from build123d import *

# Parameters (mm, degrees)
SKETCH2_R           = 7.692100041
CUT_EXTRUDE1_DEPTH  = 10
SKETCH4_W           = 16.725751486
SKETCH4_H           = 29.132579912
BOSS_EXTRUDE1_DEPTH = 15
BOSS_EXTRUDE2_START = -29.132579912
BOSS_EXTRUDE2_DEPTH = 29.132579912
CUT_EXTRUDE2_DEPTH  = 72.857514692


with BuildPart() as part:
    # Sketch1 → Revolve1 (revolve)
    with BuildSketch(Plane(origin=(0, 0, 0), x_dir=(0, 0, -1), z_dir=(1, 0, 0)), mode=Mode.PRIVATE) as revolve1_sk:
        Polygon((18, 19), (53, 19), (53, 0), (56.096816333, 0), (56.096816333, 23.355709418), (18, 23.355709418), align=None)
    revolve(revolve1_sk.sketch.rotate(Axis((0, 0, -53), (0, 0, -1)), 90), axis=Axis((0, 0, -53), (0, 0, -1)))

    # Sketch2 → Cut-Extrude1 (cut)
    with BuildSketch(Plane(origin=(0, 0, -56.096816333), x_dir=(-1, 0, 0), z_dir=(0, 0, -1))):
        Circle(SKETCH2_R)
    extrude(amount=-CUT_EXTRUDE1_DEPTH, mode=Mode.SUBTRACT)



with BuildPart() as body_2:
    # Sketch4 → Boss-Extrude1 (new body)
    with BuildSketch(Plane(origin=(0, 23.355709418, 0), x_dir=(1, 0, 0), z_dir=(0, 1, 0))):
        with Locations((0, 36.155071486)):
            Rectangle(SKETCH4_W, SKETCH4_H)
    extrude(amount=BOSS_EXTRUDE1_DEPTH)


with BuildPart() as part_1:
    add(part.part)

    add(body_2.part)  # Boss-Extrude2 merges body 2
    # Sketch5 → Boss-Extrude2 (add)
    with BuildSketch(Plane(origin=(0, 0, -50.721361442), x_dir=(-1, 0, 0), z_dir=(0, 0, -1)).offset(BOSS_EXTRUDE2_START)):
        with BuildLine():
            ThreePointArc((-15.215762233, 17.71919135), (-8.113102925, 21.901295016), (0, 23.355709418))
            Line((0, 23.355709418), (-8.362875743, 23.355709418))
            Line((-8.362875743, 23.355709418), (-9.850694039, 23.211289977))
            add(Edge.make_bspline(
                [(-9.850694039, 23.211289977), (-13.176863257, 20.945911476), (-15.215762233, 17.71919135)],
                knots=[0, 0, 0, 0.793491279, 0.793491279, 0.793491279], degree=2))
        make_face()
        with BuildLine():
            add(Edge.make_bspline(
                [(9.850694039, 23.211289977), (13.176863257, 20.945911476), (15.215762233, 17.71919135)],
                knots=[0, 0, 0, 0.793491279, 0.793491279, 0.793491279], degree=2))
            Line((9.850694039, 23.211289977), (8.362875743, 23.355709418))
            Line((8.362875743, 23.355709418), (0, 23.355709418))
            ThreePointArc((0, 23.355709418), (8.113102925, 21.901295016), (15.215762233, 17.71919135))
        make_face()
    extrude(amount=BOSS_EXTRUDE2_DEPTH)

    # Sketch6 → Cut-Extrude2 (cut, through all)
    with BuildSketch(Plane.XY):
        with BuildLine():
            Line((-16.155494421, -10), (-21.106614187, -10))
            ThreePointArc((-21.106614187, -10), (-23.355709418, 0), (-21.106614187, 10))
            Line((-21.106614187, 10), (-16.155494421, 10))
            ThreePointArc((-16.155494421, 10), (-19, 0), (-16.155494421, -10))
        make_face()
    extrude(amount=-CUT_EXTRUDE2_DEPTH, mode=Mode.SUBTRACT)


solid = part_1.part
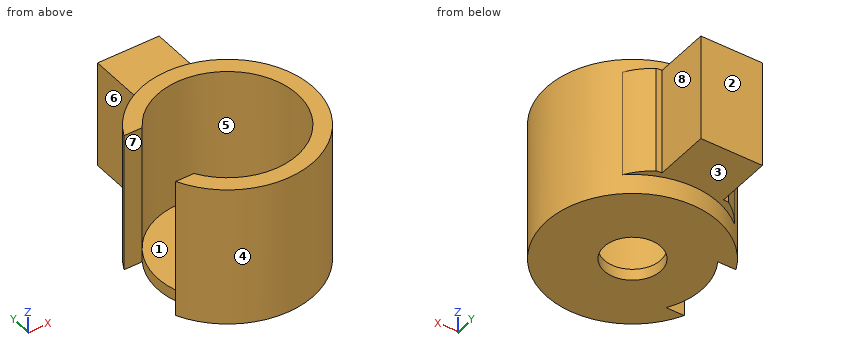
Work out the finished part from the listing and answer in its coordinate system (mm). Face numbers are marked on the shaded views. A direction names the side the tool comes from. Round coordinates to 2 decimals unless told otherwise and drop trailing zeros. Write each loop counter-clockwise with the first axis right and the second up, starting at its lowest first coordinate (ties: lowest second). Pieces come first, ordered by that corner, then holes.
1) A cutting plane is placed at C-C (z = -54). Give the vertices of the cut face in (x, y).
2) Straight lines are drawn through the part: line 1 (Y direction, x = 0.5, z = -32); line 2 (Y direction, x = 0, z = -36.5); line 3 (Z direction, x = 2, y = 13.5). For each, find the intervals that lie inside material, in ascending order.
3) A cutting plane is placed at D-D (y = -7). Give the vertices of the cut face in (x, z).
4) A cutting plane is placed at A-A (y = 0). Give the vertices of the cut face in (x, z), plus the area to 3 significant figures.
5) Given pin 1 Ø2.5 at (x, z) = (-18.5, -39) entering from -Y; pin 2 Ø5.5 at (x, z) = (-18, -43.5) entering from +Y; pin 3 Ø1 at (x, z) = (-13, -37) entering from -Y, each flat-ended and moving along its own axis, determine where each tip first touches the part or whether it passes through.
6) A cutting plane is placed at B-B (x = 0). Give the vertices of the cut face in (y, z).
7) A tool of negligible diameter and unlimited length cuts with its end or side. For the marked faces 5, 6, 7 and 8, from which of +Z, -Z, +X, -X, +Y, -Y can it reach the whole face along a straight path? Write none if from no direction.
8) The mould has two halves that part along Y. Classify the marked faces 1, 2, 3 and 4: pulls with the +Y half, pulls with the -Y half, needs draft (parallel to the pull), parting line crosses it, or undercut.
Completed:
1. outline: (-21.11, -10) arc R23.36 ccw (long way) to (-21.11, 10) - (-16.16, 10) arc R19 ccw to (-16.16, -10) - close; hole circle Ø15.38 at (0, 0)
2. line 1: y = -23.35 to -18.99, 18.99 to 38.36
2. line 2: y = -23.36 to -19, 19 to 38.36
2. line 3: z = -56.1 to -53
3. outline: (-17.66, -56.1) - (-3.19, -56.1) - (-3.19, -53) - (-17.66, -53) - close; (3.19, -56.1) - (22.28, -56.1) - (22.28, -18) - (17.66, -18) - (17.66, -53) - (3.19, -53) - close
4. outline: (-19, -56.1) - (-7.69, -56.1) - (-7.69, -53) - (-19, -53) - close; (7.69, -56.1) - (23.36, -56.1) - (23.36, -18) - (19, -18) - (19, -53) - (7.69, -53) - close
4. area: 236 mm2
5. pin 1: stops at y = -15.75
5. pin 2: stops at y = 17.69
5. pin 3: stops at y = -19.73
6. outline: (-23.36, -56.1) - (-7.69, -56.1) - (-7.69, -53) - (-19, -53) - (-19, -18) - (-23.36, -18) - close; (7.69, -56.1) - (23.36, -56.1) - (23.36, -50.72) - (38.36, -50.72) - (38.36, -21.59) - (23.36, -21.59) - (23.36, -18) - (19, -18) - (19, -53) - (7.69, -53) - close
7. face 5: +Z
7. face 6: +Z, -Z, -X, +Y
7. face 7: +Z, -Z, -X
7. face 8: +Z, -Z, +X, +Y
8. face 1: undercut
8. face 2: pulls with the +Y half
8. face 3: needs draft
8. face 4: parting line crosses it
